Here's how the part is built. I have some questions about the finished solid (model axes, mm). A direction names the side the tool comes from. Round coordinates to 2 decimals unless told otherwise and drop trailing zeros. Loops run counter-clockwise (first coordinate to the right, second up) from the corner with the lowest first, then second, coordinate; pieces in that order, holes last. Notation, with made-up numbers: M 50,67.5 L 66,67.5 A31 cw 66,99.5 Z; hole C -5,66.5 d1. An arc over 180 degrees is marked long. Answer as a JSON object with one key per item and string values.
Autodesk Inventor part; units mm, degrees
ref_plane "РабПлоскость1" through (0, 0, 0) normal (0, 0, 1) x (1, 0, 0)
ref_plane "YZ Plane" through (0, 0, 0) normal (1, 0, 0) x (0, 1, 0)
ref_plane "XZ Plane" through (0, 0, 0) normal (0, 1, 0) x (-1, 0, 0)
ref_plane "РабПлоскость1" through (0, 0, 0) normal (0, 0, 1) x (1, 0, 0)
sketch "Эскиз1" plane through (0, 0, 0) normal (0, 0, 1) x (1, 0, 0)
  circle A0 centre (22, -134.9569) radius 1.5
  circle A1 centre (22, -120.9569) radius 1.5
  circle A2 centre (35, -134.9569) radius 1.5
  circle A3 centre (35, -120.9569) radius 1.5
  line L0 (25.3767, -96.9033) -> (9.3929, -97.3164)
  line L1 (46.6684, -70.3473) -> (46.1406, -50.3565)
  line L2 (48, -90) -> (48, -70.3473)
  line L3 (17.5, -139.4569) -> (58.5, -139.4569)
  line L4 (58.5, -139.4569) -> (58.5, -116.4569)
  line L5 (58.5, -116.4569) -> (17.5, -116.4569)
  line L6 (17.5, -116.4569) -> (17.5, -139.4569)
  ellipse E0 centre (13.2497, -96.1261) end of major axis (24.2459, -95.8358) minor radius 0.1657
  point P0 (0, 0)
  point P1 (12.1906, -152.9569)
  dimension "d0" = 18
  dimension "d2" = 14
  dimension "d3" = 14
  dimension "d4" = 3
  dimension "d5" = 3
  dimension "d6" = 3
  dimension "d7" = 3
  dimension "d8" = 13
  dimension "d9" = 13
  dimension "d10" = 13
  dimension "d11" = 13
  dimension "d12" = 23
  dimension "d13" = 41
  dimension "d14" = 4.5
  dimension "d15" = 4.5
  dimension "d33" = 23.5
  dimension "d34" = 23.5
extrude "Выдавливание1" add sketch "Эскиз1" along normal blind 4 contours L6 L5 L4 L3
sketch "Эскиз2" plane through (0, 0, 4) normal (0, 0, 1) x (1, 0, 0)
  line L0 (43.5, -166.4569) -> (45.5, -166.4569)
  line L1 (45.5, -166.4569) -> (45.5, -116.4569)
  line L2 (45.5, -116.4569) -> (43.5, -116.4569)
  line L3 (43.5, -116.4569) -> (43.5, -166.4569)
  line L4 (53.5, -116.4569) -> (58.5, -116.4569)
  line L5 (58.5, -116.4569) -> (58.5, -157.4569)
  line L6 (58.5, -157.4569) -> (53.5, -157.4569)
  line L7 (53.5, -157.4569) -> (53.5, -116.4569)
  line L8 (58.5, -139.4569) -> (58.5, -116.4569)
  line L9 (58.5, -116.4569) -> (17.5, -116.4569)
  line L10 (17.5, -139.4569) -> (58.5, -139.4569)
  point P0 (0, 0)
  point P1 (58.5, -139.4569)
  point P2 (53.5, -139.4569)
  dimension "d18" = 8
  dimension "d19" = 18
  dimension "d20" = 5
  dimension "d21" = 2
  dimension "d22" = 50
extrude "Выдавливание2" add sketch "Эскиз2" along normal blind 12 contours L10 L5 L6 L7 | L7 L4 L5 L10
sketch "Эскиз3" plane through (53.5, -157.4569, 4) normal (-1, 0, 0) x (0, 0, 1)
  line L0 (0, 18) -> (0, 41)
  line L1 (0, 18) -> (0, -9) construction
  line L2 (0, -9) -> (6, -9) construction
  line L3 (6, 41) -> (6, -9) construction
  line L4 (0, 41) -> (6, 41)
  circle A0 centre (8, 8) radius 1.55
  line L5 (-4, 18) -> (0, 18)
  line L6 (12, 41) -> (12, 0)
  line L7 (0, 0) -> (12, 0)
  point P0 (-4, 157.4569)
  dimension "d26" = 3.1
  dimension "d40" = 4
  dimension "d41" = 8
extrude "Выдавливание3" cut sketch "Эскиз3" against normal through all
thread "Резьба1"
extrude "Выдавливание4" add sketch "Эскиз2" along normal blind 16 contours L3 L10 L1 L0 | L3 L2 L1 L10
sketch "Эскиз4" plane through (58.5, -139.4569, 0) normal (1, 0, 0) x (0, 0, -1)
  circle A0 centre (-12, -10) radius 1.55
  circle A1 centre (-12, -10) radius 2.05
  circle A2 centre (-12, -10) radius 8
  line L0 (-4, -18) -> (-16, -18)
  point P0 (0, 139.4569)
  dimension "d35" = 4.1
extrude "Выдавливание5" cut sketch "Эскиз4" against normal up to surface (5 mm away) contours A0 | A1
extrude "Выдавливание6" add sketch "Эскиз4" against normal up to surface (5 mm away) contours A2
sketch "Эскиз5" plane through (43.5, -166.4569, 4) normal (-1, 0, 0) x (0, 0, 1)
  circle A0 centre (8, 17) radius 2.05
  line L0 (0, 27) -> (0, 9)
  line L1 (0, 9) -> (12, 9)
  line L2 (12, 50) -> (12, 23.9282)
  line L3 (0, 50) -> (12, 50)
  line L4 (0, 27) -> (0, 50)
  arc A1 (12, 10.0718) -> (12, 23.9282) centre (8, 17) ccw
  line L5 (12, 10.0718) -> (12, 9)
  line L6 (16, 17) -> (0, 17) construction
  line L7 (16, 50) -> (16, 0)
  circle A2 centre (8, 11) radius 1.5
  circle A3 centre (8, 23) radius 1.5
  line L8 (8, 11) -> (8, 23) construction
  line L9 (0, 9) -> (3, 9)
  line L10 (3, 9) -> (3, 24)
  line L11 (3, 24) -> (0, 24)
  line L12 (0, 24) -> (0, 9)
  point P0 (-4, 166.4569)
  point P1 (8, 17)
  point P2 (0, 24)
  point P3 (3, 9)
  dimension "d49" = 3
  dimension "d50" = 3
  dimension "d52" = 15
  dimension "d53" = 6
  dimension "d54" = 5
  dimension "d55" = 15
extrude "Выдавливание7" cut sketch "Эскиз5" against normal blind 10 contours L11 L10 L1 L0 | A2 | A3
equation "\"d34\" = d33"
properties part number "робот-энкодер"
Item 1: I want a section at B-B on z = 12. List the corners of the cut face in (x, y) for me.
Solution:
{"outline": "M 43.5,-166.46 L 45.5,-166.46 L 45.5,-156.96 L 43.5,-156.96 Z; M 43.5,-153.96 L 45.5,-153.96 L 45.5,-144.96 L 43.5,-144.96 Z; M 43.5,-141.96 L 45.5,-141.96 L 45.5,-116.46 L 43.5,-116.46 Z; M 53.5,-157.46 L 58.5,-157.46 L 58.5,-151.51 L 53.5,-151.51 Z; M 53.5,-147.41 L 58.5,-147.41 L 58.5,-116.46 L 53.5,-116.46 Z"}
Item 2: We'd pull the mould along Y, two halves only. Please class faces 1 (the face through (56, -149.3, 20)), 2 (the face through (38, -128, 0)), 3 (the face through (21.805, -136.444, 1.972)), 4 (the face through (44, -166.457, 12)): +Y half, -Y half, draft (parallel to the pull), parting line (faces both ways), or undercut.
Solution:
{"face 1": "parting line", "face 2": "draft", "face 3": "undercut", "face 4": "-Y half"}
Item 3: I want a section at D-D on x = 35. List the corners of the cut face in (y, z) for me, plus the area to 3 significant figures.
Solution:
{"outline": "M -139.46,0 L -136.46,0 L -136.46,4 L -139.46,4 Z; M -133.46,0 L -122.46,0 L -122.46,4 L -133.46,4 Z; M -119.46,0 L -116.46,0 L -116.46,4 L -119.46,4 Z", "area": "68.0 mm2"}
Item 4: For P1, Ø2.5, axis at x = 57, y = -134, coming from the +Z side; P2, Ø5, axis at x = 46.5, y = -158.5, coming from the -Z side; P3, Ø1.6, axis at x = 45, y = -147, coming from the -Z side; P4, Ø2.5, axis at x = 35, y = -134.96, coming from the -Z side, each with a flat end and sliding along its axis, tell me the tip position at first contact or that it passes through.
Solution:
{"P1": "stops at z = 16", "P2": "stops at z = 4", "P3": "stops at z = 7", "P4": "passes through"}
Item 5: For faces 5 (the face through (56, -129, 16)), 6 (the face through (30, -128, 4)), 7 (the face through (56, -148, 4)), which set-ups out of +Z, -Z, +X, -X, +Y, -Y let a thin tool reach every point of the face, with its end or its side?
Solution:
{"face 5": "+Z, +X, +Y", "face 6": "+Z, -X, +Y, -Y", "face 7": "-Z, +X, -X, -Y"}
Item 6: I want a section at C-C on y = -141. List the corners of the cut face in (x, z) for me.
Solution:
{"outline": "M 43.5,4 L 45.5,4 L 45.5,20 L 43.5,20 Z; M 53.5,4 L 58.5,4 L 58.5,16 L 53.5,16 Z"}
Item 7: If I drill on L1, parallel to Y at x = 22, z = 1.8; L2, parallel to Y at x = 44.4, z = 12; L3, parallel to X at y = -148.5, z = 15.5, over which ranges is the centre line in solid material (lowest first)? Write a range as from..to.
Solution:
{"L1": "y = -139.46..-136.46, -133.46..-122.46, -119.46..-116.46", "L2": "y = -166.46..-156.96, -153.96..-144.96, -141.96..-116.46", "L3": "x = 43.5..45.5, 53.5..58.5"}
Item 8: I want a section at A-A on z = 9.25. List the corners of the cut face in (x, y) for me.
Solution:
{"outline": "M 43.5,-166.46 L 45.5,-166.46 L 45.5,-116.46 L 43.5,-116.46 Z; M 53.5,-157.46 L 58.5,-157.46 L 58.5,-116.46 L 53.5,-116.46 Z"}
